Design review of the part built by this model. Coordinates are the model's own, in mm. A direction names the side the tool comes from. Give positions to 0.01 mm unless a question says otherwise; leave off trailing zeros. Write each loop counter-clockwise with the first axis right and the second up, starting at its lowest first coordinate (ties: lowest second). Pieces come first, ordered by that corner, then holes. Notation, with made-up numbers: M -13.75,31.25 L 17.25,31.25 A32 ccw 17.25,60.25 Z; hole C 66,36.5 d7. An arc over 180 degrees is marked long. Use a Markdown table: item, result. Add a question column.
```python
from build123d import *

# Parameters (mm, degrees)
F0_W     = 25.4
F0_H     = 106.68
F1_DEPTH = 12.7
F3_DEPTH = 27.94
F4_R     = 3.175
F5_DEPTH = 25.4
F6_R     = 5.55625
F7_DEPTH = 25.4
F9_DEPTH = 25.4
F10_SIZE = 0.508
F11_SIZE = 0.254
F12_R    = 9.525
F13_SIZE = 0.254


with BuildPart() as f1:
    # F0 (on Top) → F1 (new body)
    with BuildSketch(Plane.XY):
        with Locations((12.7, 53.34)):
            Rectangle(F0_W, F0_H)
    extrude(amount=F1_DEPTH)

    # F2 (on Right) → F3 (cut)
    with BuildSketch(Plane.YZ):
        with BuildLine():
            ThreePointArc((21.59, 7.14375), (21.8224839924, 6.5824839924), (22.38375, 6.35))
            Line((22.38375, 6.35), (84.29625, 6.35))
            ThreePointArc((84.29625, 6.35), (84.8575160076, 6.5824839924), (85.09, 7.14375))
            Line((85.09, 7.14375), (85.09, 19.05))
            Line((85.09, 19.05), (21.59, 19.05))
            Line((21.59, 19.05), (21.59, 7.14375))
        make_face()
    extrude(amount=F3_DEPTH, mode=Mode.SUBTRACT)

    # F4 (on Top) → F5 (cut)
    with BuildSketch(Plane.XY):
        with Locations((12.7, 80.8355)):
            Circle(F4_R)
        with Locations((12.7, 25.8445)):
            Circle(F4_R)
    extrude(amount=F5_DEPTH, mode=Mode.SUBTRACT)

    # F6 (on Top) → F7 (cut)
    with BuildSketch(Plane.XY):
        with Locations((12.7, 93.98)):
            Circle(F6_R)
        with Locations((12.7, 12.7)):
            Circle(F6_R)
    extrude(amount=F7_DEPTH, mode=Mode.SUBTRACT)

    # F8 (on Top) → F9 (cut)
    with BuildSketch(Plane.XY):
        with BuildLine():
            Line((14.2875, 72.39), (11.1125, 72.39))
            ThreePointArc((11.1125, 72.39), (6.6223719395, 70.5301280605), (4.7625, 66.04))
            Line((4.7625, 66.04), (4.7625, 40.64))
            ThreePointArc((4.7625, 40.64), (6.6223719395, 36.1498719395), (11.1125, 34.29))
            Line((11.1125, 34.29), (14.2875, 34.29))
            ThreePointArc((14.2875, 34.29), (18.7776280605, 36.1498719395), (20.6375, 40.64))
            Line((20.6375, 40.64), (20.6375, 66.04))
            ThreePointArc((20.6375, 66.04), (18.7776280605, 70.5301280605), (14.2875, 72.39))
        make_face()
    extrude(amount=F9_DEPTH, mode=Mode.SUBTRACT)

    # F10
    f10_edges = [f1.edges().sort_by_distance(p)[0] for p in [
        (7.14375, 12.7, 0),
        (7.14375, 93.98, 0),
        (9.525, 80.8355, 0),
        (9.525, 25.8445, 0),
        (7.14375, 93.98, 12.7),
        (7.14375, 12.7, 12.7),
    ]]
    chamfer(f10_edges, length=F10_SIZE)

    # F11
    f11_edges = [f1.edges().sort_by_distance(p)[0] for p in [
        (4.7625, 53.34, 0),
        (20.6375, 53.34, 6.35),
    ]]
    chamfer(f11_edges, length=F11_SIZE)

    # F12
    f12_edges = [f1.edges().sort_by_distance(p)[0] for p in [
        (25.4, 0, 6.35),
        (0, 0, 6.35),
        (25.4, 106.68, 6.35),
        (0, 106.68, 6.35),
    ]]
    fillet(f12_edges, radius=F12_R)

    # F13
    f13_edges = [f1.edges().sort_by_distance(p)[0] for p in [
        (0, 53.34, 0),
    ]]
    chamfer(f13_edges, length=F13_SIZE)


solid = f1.part
```
(1) Add section C-C on y = 46.5. Give the boundary of the cut face in (x, z).
(2) Machinability: for faces 4 (the cylindrical face through (6.573, 36.2, 3.134)), 5 (the conical face through (18.916, 70.568, 0.129)), 6 (the conical face through (18.818, 70.671, 6.225)), 7 (the flat face through (13, 85.09, 10)), which of the approach directions +Z, -Z, +X, -X, +Y, -Y give a long, thin tool a straight path to every point of the face, cutting with its end or side? Answer none if there is none.
(3) Add section A-A on y = 12.7. Give the boundary of the cut face in (x, z).
(4) Add section B-B on z = 8.5. Give the number of separate pieces and of enclosed holes in the cut face, then the cut area to 3 significant figures.
(5) Wall thickness on L1, parallel to Y at x = 12.7, z = 3.25; L2, parallel to X at y = 42, z = 5.25; L3, parallel to Y at x = 14.25, z = 3: over which ranges is each line inside the solid? List them lowest first.
(6) The part is to be moulded in two halves that separate along Y. For faces 1 (the conical face through (2.952, 2.806, 0.129)), 2 (the flat face through (25.4, 53, 4)), 3 (the flat face through (4.762, 54, 3)), say which applies: released by +Y, released by -Y, zero draft, split by the parting line, or undercut.
(7) For pin 1 (3 mm diameter, centred on x = 7.5, z = 4, fed in from -Y); pin 2 (7.5 mm diameter, centred on x = 12.7, y = 80.84, fed in from +Z); pin 3 (4.5 mm diameter, centred on x = 19, z = 9, fed in from +Y), all flat-tipped, find the tip position at first contact; note any pin that passes through.
From the geometry:
| question | item | result |
|---|---|---|
| 1 | outline | M 0,0.25 L 0.25,0 L 4.51,0 L 4.76,0.25 L 4.76,6.1 L 4.51,6.35 L 0,6.35 Z; M 20.64,0.25 L 20.89,0 L 25.15,0 L 25.4,0.25 L 25.4,6.35 L 20.89,6.35 L 20.64,6.1 Z |
| 2 | face 4 | +Z, -Z |
| 2 | face 5 | -Z |
| 2 | face 6 | +Z |
| 2 | face 7 | +Z, +X, -X |
| 3 | outline | M 0,0.25 L 0.25,0 L 6.64,0 L 7.14,0.51 L 7.14,12.19 L 6.64,12.7 L 0,12.7 Z; M 18.26,0.51 L 18.76,0 L 25.15,0 L 25.4,0.25 L 25.4,12.7 L 18.76,12.7 L 18.26,12.19 Z |
| 4 | separate pieces | 2 |
| 4 | enclosed holes | 2 |
| 4 | area | 825 mm^2 |
| 5 | L1 | y = 0 to 7.14, 18.26 to 22.67, 29.02 to 34.29, 72.39 to 77.66, 84.01 to 88.42, 99.54 to 106.68 |
| 5 | L2 | x = 0 to 4.76, 20.64 to 25.4 |
| 5 | L3 | y = 0 to 7.36, 18.04 to 23.07, 28.62 to 34.29, 72.39 to 78.06, 83.61 to 88.64, 99.32 to 106.68 |
| 6 | face 1 | released by -Y |
| 6 | face 2 | zero draft |
| 6 | face 3 | undercut |
| 7 | pin 1 | stops at y = 0.01 |
| 7 | pin 2 | stops at z = 6.41 |
| 7 | pin 3 | stops at y = 106.64 |
